from build123d import *

# Parameters (mm, degrees)
F0_R     = 11
F1_DEPTH = 2
F2_R     = 5
F3_DEPTH = 1
F4_R     = 3.95
F5_DEPTH = 3
F6_R     = 3
F7_DEPTH = 3
F8_SIZE  = 0.5
F9_R     = 0.3


with BuildPart() as f1:
    # F0 (on Top) → F1 (new body)
    with BuildSketch(Plane.XY):
        Circle(F0_R)
    extrude(amount=F1_DEPTH)

    # F2 (on face) → F3 (join)
    with BuildSketch(Plane.XY.offset(2)):
        Circle(F2_R)
    extrude(amount=F3_DEPTH)

    # F4 (on face) → F5 (join)
    with BuildSketch(Plane.XY.offset(3)):
        Circle(F4_R)
    extrude(amount=F5_DEPTH)

    # F6 (on face) → F7 (cut)
    with BuildSketch(Plane.XY.offset(6)):
        Circle(F6_R)
    extrude(amount=-F7_DEPTH, mode=Mode.SUBTRACT)

    # F8
    f8_edges = [f1.edges().sort_by_distance(p)[0] for p in [
        (-3.95, 0, 6),
    ]]
    chamfer(f8_edges, length=F8_SIZE)

    # F9
    f9_edges = [f1.edges().sort_by_distance(p)[0] for p in [
        (-3.95, 0, 5.5),
    ]]
    fillet(f9_edges, radius=F9_R)


solid = f1.part
Part model, mm, in its own coordinate system. A direction names the side the tool comes from. Round coordinates to 2 decimals unless told otherwise and drop trailing zeros. Write each loop counter-clockwise with the first axis right and the second up, starting at its lowest first coordinate (ties: lowest second). Pieces come first, ordered by that corner, then holes. Notation, with made-up numbers: M 76,67 L 126,67 A11 ccw 126,79 Z; hole C 10,28 d3. An arc over 180 degrees is marked long. Return JSON: item names as keys, results as strings. Group by question number.
(1) Saw through at B-B on x = 4.25. Write the cut outline in (y, z), then the cut area to 3 significant figures.
(2) Two-plate mould, pull along X, no slides. Class faces 3 (the face through (3.65, -1.51, 4.17)), 4 (the face through (-3, 0, 5)), 5 (the face through (4, 2, 3)): +X half, -X half, draft (parallel to the pull), parting line (faces both ways), or undercut.
(3) Saw through at C-C on y = -6. Write the cut outline in (x, z), then the cut area to 3 significant figures.
(4) Drill centre lines: probe 1 along Y at (x, z) = (0, 5.15); probe 2 along Z at (x, y) = (7.5, -3.25); probe 3 along X at (y, z) = (-1.5, 4.5). Where is each one in solid material? Low to high.
(5) Saw through at D-D on x = 7.5. Write the cut outline in (y, z).
(6) Pin check, flat tips, straight feed: pin 1 Ø1.5 at (x, y) = (-1.5, -5) entering from +Z; pin 2 Ø1.5 at (y, z) = (-6.5, 3) entering from +X. Stop position of each tip, or through.
(7) Which spindle directions (+Z, -Z, +X, -X, +Y, -Y) get a long thin tool onto all of the face, cutting with end or side? Do faces 1 (the face through (0, 0, 0)), 2 (the face through (2, -5, 2)). Say none if no direction does.
(8) Saw through at A-A on z = 4. Write the cut outline in (x, y), then the cut area to 3 significant figures.
Returned:
{
 "1": {"outline": "M -10.15,0 L 10.15,0 L 10.15,2 L 2.63,2 L 2.63,3 L -2.63,3 L -2.63,2 L -10.15,2 Z", "area": "45.9 mm²"},
 "2": {"face 3": "parting line", "face 4": "undercut", "face 5": "draft"},
 "3": {"outline": "M -9.22,0 L 9.22,0 L 9.22,2 L -9.22,2 Z", "area": "36.9 mm²"},
 "4": {"probe 1": "-3.95 to -3, 3 to 3.95", "probe 2": "0 to 2", "probe 3": "-3.65 to -2.6, 2.6 to 3.65"},
 "5": {"outline": "M -8.05,0 L 8.05,0 L 8.05,2 L -8.05,2 Z"},
 "6": {"pin 1": "z = 3", "pin 2": "through"},
 "7": {"face 1": "-Z, +X, -X, +Y, -Y", "face 2": "+Z"},
 "8": {"outline": "C 0,0 d7.9; hole C 0,0 d6", "area": "20.7 mm²"}
}
